Here's how the part is built. I have some questions about the finished solid (model axes, mm). A direction names the side the tool comes from. Round coordinates to 2 decimals unless told otherwise and drop trailing zeros. Write each loop counter-clockwise with the first axis right and the second up, starting at its lowest first coordinate (ties: lowest second). Pieces come first, ordered by that corner, then holes. Notation, with made-up numbers: (4, 25.25) - (56, 25.25) arc R27 cw to (56, 51.25) - close; hole circle Ø8 at (2.25, -22). An arc over 180 degrees is marked (long way). Return JSON: item names as keys, results as strings. Group by question number.
```python
from build123d import *

# Parameters (mm, degrees)
SKETCH1_R           = 75
BOSS_EXTRUDE1_DEPTH = 30
SKETCH2_R           = 2.5
CUT_EXTRUDE1_DEPTH  = 31
SHELL1_T            = -10


with BuildPart() as part:
    # Sketch1 → Boss-Extrude1 (new body)
    with BuildSketch(Plane.XY):
        Circle(SKETCH1_R)
    extrude(amount=BOSS_EXTRUDE1_DEPTH)

    # Sketch2 → Cut-Extrude1 (cut, through all)
    with BuildSketch(Plane(origin=(0, 0, 0), x_dir=(-1, 0, 0), z_dir=(0, 0, -1))):
        Circle(SKETCH2_R)
    extrude(amount=-CUT_EXTRUDE1_DEPTH, mode=Mode.SUBTRACT)

    # Shell1
    shell1_openings = [part.faces().sort_by_distance(p)[0] for p in [
        (-2.5, 0, 0),
    ]]
    offset(amount=SHELL1_T, openings=shell1_openings, kind=Kind.INTERSECTION)


solid = part.part
```
1) For faces 1 (the cylindrical face through (62, 19.52, 9.86)), 2 (the flat face through (0, -3, 0)), which set-ups out of +Z, -Z, +X, -X, +Y, -Y let a thin tool reach every point of the face, with its end or its side?
2) Imagine slicing it at C-C (z = 2.5). Please give me the cut outline in (x, y), plus the area to 3 significant figures.
3) I need wall thicknesses on line 1 along Y through (x, z) = (0, 10); line 2 along X through (y, z) = (4.5, 5); line 3 along Z through (x, y) = (-19, 20.5). Which ranges of each line are inside material? Lowest first, please.
4) If we mould it in two halves opening along X, with no side actions, what happens to faces 3 (the cylindrical face through (-11.923, 3.755, 9.86)), 4 (the flat face through (-23, 61, 0)), 5 (the cylindrical face through (-9.764, 74.362, 14.79)), 6 (the flat face through (14, 1, 20))? For each: released by +X, released by -X, zero draft, split by the parting line, or undercut.
5) Will these pins go through, and if not, where does the flat tip stop? pin 1 Ø4.5 at (x, y) = (0, 0) entering from -Z; pin 2 Ø2 at (y, z) = (12, 17.5) entering from +X; pin 3 Ø2 at (y, z) = (5, 12.5) entering from +X; pin 4 Ø12 at (x, z) = (-48.5, 7) entering from -Y.
6) Imagine slicing it at A-A (x = 0). Please give me the cut outline in (y, z), plus the area to 3 significant figures.
7) Imagine slicing it at D-D (x = -60). Please give me the cut outline in (y, z), plus the area to 3 significant figures.
Results found:
{
 "1": {"face 1": "-Z", "face 2": "-Z, +X, -X, +Y, -Y"},
 "2": {"outline": "circle Ø150 at (0, 0); circle Ø25 at (0, 0); hole circle Ø130 at (0, 0); hole circle Ø5 at (0, 0)", "area": "4,870 mm²"},
 "3": {"line 1": "y = -75 to -65, -12.5 to -2.5, 2.5 to 12.5, 65 to 75", "line 2": "x = -74.86 to -64.84, -11.66 to 11.66, 64.84 to 74.86", "line 3": "z = 20 to 30"},
 "4": {"face 3": "undercut", "face 4": "zero draft", "face 5": "split by the parting line", "face 6": "undercut"},
 "5": {"pin 1": "passes through", "pin 2": "stops at x = 74.19", "pin 3": "stops at x = 74.89", "pin 4": "stops at y = -61.8"},
 "6": {"outline": "(-75, 0) - (-65, 0) - (-65, 20) - (-12.5, 20) - (-12.5, 0) - (-2.5, 0) - (-2.5, 30) - (-75, 30) - close; (2.5, 0) - (12.5, 0) - (12.5, 20) - (65, 20) - (65, 0) - (75, 0) - (75, 30) - (2.5, 30) - close", "area": "2,250 mm²"},
 "7": {"outline": "(-45, 0) - (-25, 0) - (-25, 20) - (25, 20) - (25, 0) - (45, 0) - (45, 30) - (-45, 30) - close", "area": "1,700 mm²"}
}
